Autodesk Inventor part; units mm, degrees
ref_plane "socket_XY" through (3.9116, 0, 0) normal (0, 1, 0) x (1, 0, 0)
ref_plane "socket_YZ" through (3.9116, 0, 0) normal (1, 0, 0) x (0, 0, -1)
ref_plane "socket_ZX" through (3.9116, 0, 0) normal (0, 0, -1) x (0, 1, 0)
sketch "Sketch_17" plane through (0, 0, 0) normal (0, 1, 0) x (-1, 0, 0)
  line L0 (-0.254, -0.635) -> (-0.254, 0.635)
  line L1 (-0.254, 0.635) -> (-7.5692, 0.635)
  line L2 (-7.5692, 0.635) -> (-7.5692, -0.635)
  line L3 (-7.5692, -0.635) -> (-0.254, -0.635)
extrude "Extrusion1" add sketch "Sketch_17" along normal blind 2.54
sketch "Sketch_3" plane through (0, 0, 0) normal (0, 1, 0) x (-1, 0, 0)
  line L0 (0, 0.635) -> (-0.1701, 1.27)
  line L1 (-0.1701, 1.27) -> (-2.4376, 1.27)
  line L2 (-2.4376, 1.27) -> (-2.6077, 0.635)
  line L3 (-2.6077, 0.635) -> (-2.6077, -0.635)
  line L4 (-2.6077, -0.635) -> (-2.4376, -1.27)
  line L5 (-2.4376, -1.27) -> (-0.1701, -1.27)
  line L6 (-0.1701, -1.27) -> (0, -0.635)
  line L7 (0, -0.635) -> (0, 0.635)
extrude "Extrusion2" add sketch "Sketch_3" along normal blind 2.54
pattern_linear "Rectangular Pattern1" count 3 spacing 2.6077 along (1, 0, 0) of "Extrusion2"
sketch "Sketch3" plane through (0, 0, 0) normal (0, -1, 0) x (1, 0, 0)
  point P0 (1.3716, 0)
hole "Hole1" at (1.3716, 0, 0) direction (0, 1, 0) diameter 1.3208 depth 2.54
pattern_linear "Rectangular Pattern2" count 3 spacing 2.54 along (1, 0, 0) of "Hole1"
sketch "Sketch_7" plane through (0, 2.54, 0) normal (0, 1, 0) x (1, 0, 0)
  circle A0 centre (1.3716, 0) radius 0.889
extrude "Extrusion3" cut sketch "Sketch_7" against normal blind 0.762
pattern_linear "Rectangular Pattern3" count 3 spacing 2.54 along (1, 0, 0) of "Extrusion3"
ref_plane "socket_XY" through (3.9116, 0, 0) normal (0, 1, 0) x (1, 0, 0)
ref_plane "socket_YZ" through (3.9116, 0, 0) normal (1, 0, 0) x (0, 0, -1)
ref_plane "socket_ZX" through (3.9116, 0, 0) normal (0, 0, -1) x (0, 1, 0)
ref_plane "to_pin_1_XY" through (1.3716, 2.7432, 0) normal (0, 1, 0) x (1, 0, 0)
ref_plane "to_pin_1_YZ" through (1.3716, 2.7432, 0) normal (1, 0, 0) x (0, 0, -1)
ref_plane "to_pin_1_ZX" through (1.3716, 2.7432, 0) normal (0, 0, -1) x (0, 1, 0)
ref_plane "to_pin_2_XY" through (3.9116, 2.7432, 0) normal (0, 1, 0) x (1, 0, 0)
ref_plane "to_pin_2_YZ" through (3.9116, 2.7432, 0) normal (1, 0, 0) x (0, 0, -1)
ref_plane "to_pin_2_ZX" through (3.9116, 2.7432, 0) normal (0, 0, -1) x (0, 1, 0)
ref_plane "to_pin_3_XY" through (6.4516, 2.7432, 0) normal (0, 1, 0) x (1, 0, 0)
ref_plane "to_pin_3_YZ" through (6.4516, 2.7432, 0) normal (1, 0, 0) x (0, 0, -1)
ref_plane "to_pin_3_ZX" through (6.4516, 2.7432, 0) normal (0, 0, -1) x (0, 1, 0)
ref_plane "to_pin2_1_XY" through (1.3716, 2.7432, 0) normal (0, 1, 0) x (1, 0, 0)
ref_plane "to_pin2_1_YZ" through (1.3716, 2.7432, 0) normal (1, 0, 0) x (0, 0, -1)
ref_plane "to_pin2_1_ZX" through (1.3716, 2.7432, 0) normal (0, 0, -1) x (0, 1, 0)
ref_plane "to_pin2_2_XY" through (3.9116, 2.7432, 0) normal (0, 1, 0) x (1, 0, 0)
ref_plane "to_pin2_2_YZ" through (3.9116, 2.7432, 0) normal (1, 0, 0) x (0, 0, -1)
ref_plane "to_pin2_2_ZX" through (3.9116, 2.7432, 0) normal (0, 0, -1) x (0, 1, 0)
ref_plane "to_pin2_3_XY" through (6.4516, 2.7432, 0) normal (0, 1, 0) x (1, 0, 0)
ref_plane "to_pin2_3_YZ" through (6.4516, 2.7432, 0) normal (1, 0, 0) x (0, 0, -1)
ref_plane "to_pin2_3_ZX" through (6.4516, 2.7432, 0) normal (0, 0, -1) x (0, 1, 0)
properties part number "TS-103-G-A_socket"
Here's how the part is built. I have some questions about the finished solid (model axes, mm). A direction names the side the tool comes from. Coordinates: 2 decimals unless noted, no trailing zeros. Write each loop counter-clockwise with the first axis right and the second up, starting at its lowest first coordinate (ties: lowest second). Pieces come first, ordered by that corner, then holes.
1) I'm going to push flat-ended pins straight in: pin 1 (1.4 mm diameter, centred on x = 4, z = 0.5, fed in from +Y); pin 2 (1.4 mm diameter, centred on x = 1.5, z = 0, fed in from +Y). Where does each tip first touch, or does it pass through?
Filled in:
pin 1: stops at y = 2.54
pin 2: stops at y = 1.78
2) If we section it at D-D (z = 0.8): List the corners of the cut face in (x, y) for me, plus the area to 3 significant figures.
Filled in:
outline: (0.04, 0) - (2.56, 0) - (2.56, 2.54) - (1.76, 2.54) - (1.76, 1.78) - (0.98, 1.78) - (0.98, 2.54) - (0.04, 2.54) - close; (2.65, 0) - (5.17, 0) - (5.17, 2.54) - (4.3, 2.54) - (4.3, 1.78) - (3.52, 1.78) - (3.52, 2.54) - (2.65, 2.54) - close; (5.26, 0) - (7.78, 0) - (7.78, 2.54) - (6.84, 2.54) - (6.84, 1.78) - (6.06, 1.78) - (6.06, 2.54) - (5.26, 2.54) - close
area: 17.4 mm2
3) If we section it at B-B (x = 3.5): List the corners of the cut face in (y, z) for me, plus the area to 3 significant figures.
Filled in:
outline: (0, -1.27) - (2.54, -1.27) - (2.54, -0.79) - (1.78, -0.79) - (1.78, -0.52) - (0, -0.52) - close; (0, 0.52) - (1.78, 0.52) - (1.78, 0.79) - (2.54, 0.79) - (2.54, 1.27) - (0, 1.27) - close
area: 3.41 mm2
4) Which directions (+Z, -Z, +X, -X, +Y, -Y) give clear straight access to the entire face, cutting with the end or side of a thin tool? Please do faces 5 (the face through (0.666, 2.164, 0.541)), 6 (the face through (1, 1, 1.27)).
Filled in:
face 5: +Y
face 6: +Z, +X, -X, +Y, -Y
5) If I drill on line 1 (X direction, y = 0.5, z = 0); line 2 (X direction, y = 2.15, z = 0); line 3 (Z direction, x = 6.5, y = 1.95), over which ranges is the centre line in solid material (lowest first)?
Filled in:
line 1: x = 0 to 0.71, 2.03 to 3.25, 4.57 to 5.79, 7.11 to 7.82
line 2: x = 0 to 0.48, 2.26 to 3.02, 4.8 to 5.56, 7.34 to 7.82
line 3: z = -1.27 to -0.89, 0.89 to 1.27
6) If we section it at A-A (z = 0): List the corners of the cut face in (x, y) for me, plus the area to 3 significant figures.
Filled in:
outline: (0, 0) - (0.71, 0) - (0.71, 1.78) - (0.48, 1.78) - (0.48, 2.54) - (0, 2.54) - close; (2.03, 0) - (3.25, 0) - (3.25, 1.78) - (3.02, 1.78) - (3.02, 2.54) - (2.26, 2.54) - (2.26, 1.78) - (2.03, 1.78) - close; (4.57, 0) - (5.79, 0) - (5.79, 1.78) - (5.56, 1.78) - (5.56, 2.54) - (4.8, 2.54) - (4.8, 1.78) - (4.57, 1.78) - close; (7.11, 0) - (7.82, 0) - (7.82, 2.54) - (7.34, 2.54) - (7.34, 1.78) - (7.11, 1.78) - close
area: 8.76 mm2
7) Thinking about a two-plate mould opening in X: for faces 1 (the face through (5.563, 2.164, -0.039)), 2 (the face through (3.023, 2.164, -0.039)), 3 (the face through (4, 1, -1.27)), 4 (the face through (7.823, 1, 0)), which applies, +X half, -X half, draft (parallel to the pull), parting line (faces both ways), or undercut?
Filled in:
face 1: undercut
face 2: undercut
face 3: draft
face 4: +X half
8) If we section it at C-C (y = 2.3): List the corners of the cut face in (x, z) for me (1 decimal).
Filled in:
outline: (0, -0.6) - (0.2, -1.3) - (2.4, -1.3) - (2.6, -0.6) - (2.8, -1.3) - (5, -1.3) - (5.2, -0.6) - (5.4, -1.3) - (7.7, -1.3) - (7.8, -0.6) - (7.8, 0.6) - (7.7, 1.3) - (5.4, 1.3) - (5.2, 0.6) - (5, 1.3) - (2.8, 1.3) - (2.6, 0.6) - (2.4, 1.3) - (0.2, 1.3) - (0, 0.6) - close; hole circle Ø1.8 at (1.4, 0); hole circle Ø1.8 at (3.9, 0); hole circle Ø1.8 at (6.5, 0)
